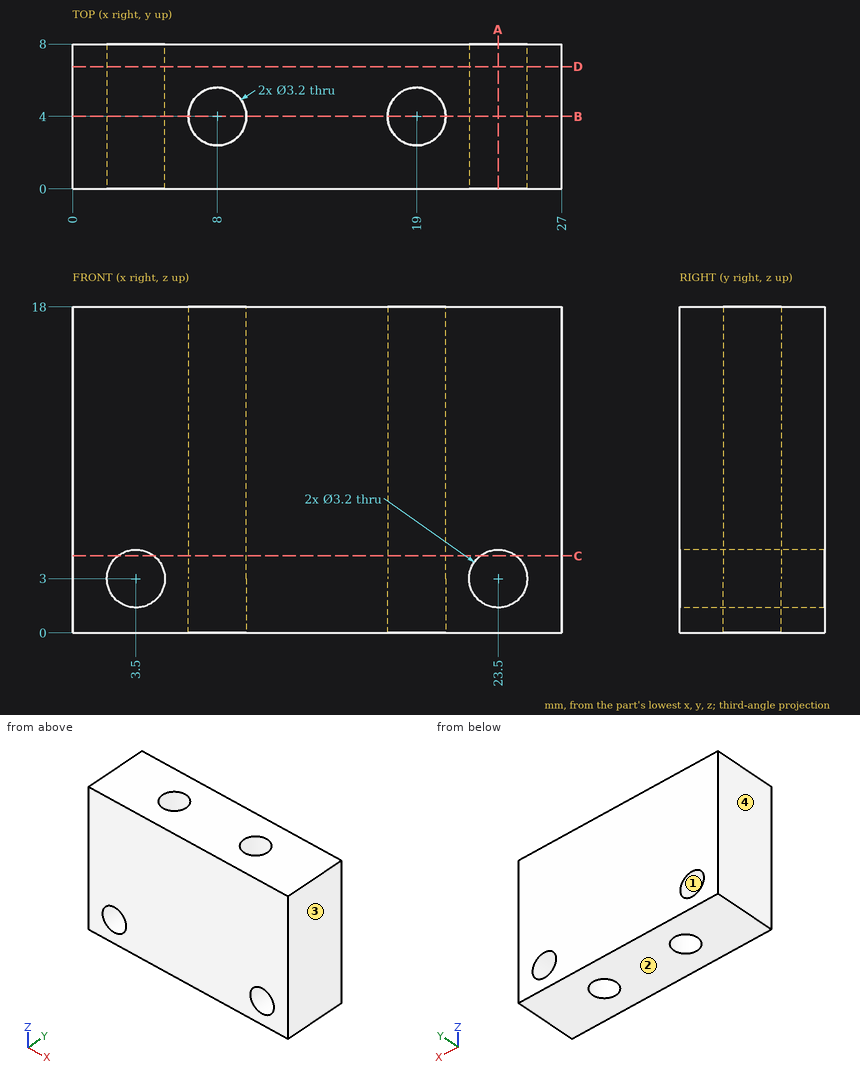
Geometry check sheet. Reference: drawing and pictorial views, mm from the part's lowest x, y, z. Give positions to 0.01 mm unless a question says otherwise; leave off trailing zeros. Order: outer loops, then holes, each group sorted by start corner. A loop starts at its lowest first (then second) coordinate and runs counter-clockwise, first axis right, second up. Notation, with made-up numbers: M 36.25,-38 L 75.25,-38 A12 cw 75.25,-28 Z; hole C -11.5,63 d2. An arc over 180 degrees is marked long. Answer as a JSON object with one key per item and string values. Group by question number.
1) Cross-section at A-A (x = 23.5). Enter the section's corners in (y, z).
2) Scan lines: line 1 along X through (y, z) = (4, 9); line 2 along Z through (x, y) = (23.5, 1.5); line 3 along Y through (x, z) = (8, 8.75). Record each from-to range of solid material in increasing order. Write a range as [from, to].
3) Cross-section at D-D (y = 6.75). Enter the section's corners in (x, z), then the cut area to 3 significant figures.
4) Cross-section at C-C (z = 4.25). Enter the section's corners in (x, y).
5) Cross-section at B-B (y = 4). Enter the section's corners in (x, z).
6) Mould release check, pull along X, two halves, no side actions. Record for the marked faces 1, 2, 3 and 4: released by +X, released by -X, zero draft, split by the parting line, or undercut.
Result sheet:
{
 "1": {"outline": "M 0,0 L 8,0 L 8,1.4 L 0,1.4 Z; M 0,4.6 L 8,4.6 L 8,18 L 0,18 Z"},
 "2": {"line 1": "x = [0, 6.4], [9.6, 17.4], [20.6, 27]", "line 2": "z = [0, 1.4], [4.6, 18]", "line 3": "y = [0, 2.4], [5.6, 8]"},
 "3": {"outline": "M 0,0 L 27,0 L 27,18 L 0,18 Z; hole C 3.5,3 d3.2; hole C 23.5,3 d3.2", "area": "470 mm2"},
 "4": {"outline": "M 0,0 L 2.5,0 L 2.5,8 L 0,8 Z; M 4.5,0 L 22.5,0 L 22.5,8 L 4.5,8 Z; M 24.5,0 L 27,0 L 27,8 L 24.5,8 Z; hole C 8,4 d3.2; hole C 19,4 d3.2"},
 "5": {"outline": "M 0,0 L 6.4,0 L 6.4,18 L 0,18 Z; M 9.6,0 L 17.4,0 L 17.4,18 L 9.6,18 Z; M 20.6,0 L 27,0 L 27,18 L 20.6,18 Z; hole C 3.5,3 d3.2; hole C 23.5,3 d3.2"},
 "6": {"face 1": "undercut", "face 2": "zero draft", "face 3": "released by +X", "face 4": "released by -X"}
}
